```python
from build123d import *

# Parameters (mm, degrees)
F1_DEPTH = 38.1
F2_DEPTH = 2
F3_DEPTH = 12.7


with BuildPart() as f1:
    # F0 (on Top) → F1 (new body)
    with BuildSketch(Plane.XY):
        with BuildLine():
            Line((-57.138, -76.9493), (-18.130362, -76.9493))
            Line((-18.130362, -76.9493), (57.138, -76.9493))
            ThreePointArc((57.138, -76.9493), (71.1472, -71.1465), (76.95, -57.1373))
            Line((76.95, -57.1373), (76.95, 57.1373))
            ThreePointArc((76.95, 57.1373), (71.1472, 71.1465), (57.138, 76.9493))
            Line((57.138, 76.9493), (-57.138, 76.9493))
            ThreePointArc((-57.138, 76.9493), (-71.1472, 71.1465), (-76.95, 57.1373))
            Line((-76.95, 57.1373), (-76.95, -57.1373))
            ThreePointArc((-76.95, -57.1373), (-71.1472, -71.1465), (-57.138, -76.9493))
        make_face()
        with BuildLine():
            Line((-56.388, 76.2), (56.388, 76.2))
            ThreePointArc((56.388, 76.2), (70.3972, 70.3972), (76.2, 56.388))
            Line((76.2, 56.388), (76.2, -56.388))
            ThreePointArc((76.2, -56.388), (70.3972, -70.3972), (56.388, -76.2))
            Line((56.388, -76.2), (-18.130362, -76.2))
            Line((-18.130362, -76.2), (-56.388, -76.2))
            ThreePointArc((-56.388, -76.2), (-70.3972, -70.3972), (-76.2, -56.388))
            Line((-76.2, -56.388), (-76.2, 56.388))
            ThreePointArc((-76.2, 56.388), (-70.3972, 70.3972), (-56.388, 76.2))
        make_face(mode=Mode.SUBTRACT)
    extrude(amount=F1_DEPTH)

    # F0 (on Top) → F2 (join)
    with BuildSketch(Plane.XY):
        with BuildLine():
            ThreePointArc((76.2, 56.388), (70.3972, 70.3972), (56.388, 76.2))
            Line((56.388, 76.2), (-56.388, 76.2))
            ThreePointArc((-56.388, 76.2), (-70.3972, 70.3972), (-76.2, 56.388))
            Line((-76.2, 56.388), (-76.2, -56.388))
            ThreePointArc((-76.2, -56.388), (-70.3972, -70.3972), (-56.388, -76.2))
            Line((-56.388, -76.2), (-18.130362, -76.2))
            Line((-18.130362, -76.2), (56.388, -76.2))
            ThreePointArc((56.388, -76.2), (70.3972, -70.3972), (76.2, -56.388))
            Line((76.2, -56.388), (76.2, 56.388))
        make_face()
    extrude(amount=F2_DEPTH)

    # F0 (on Top) → F3 (join)
    with BuildSketch(Plane.XY):
        with BuildLine():
            Line((-57.138, -76.9493), (-18.130362, -76.9493))
            Line((-18.130362, -76.9493), (57.138, -76.9493))
            ThreePointArc((57.138, -76.9493), (71.1472, -71.1465), (76.95, -57.1373))
            Line((76.95, -57.1373), (76.95, 57.1373))
            ThreePointArc((76.95, 57.1373), (71.1472, 71.1465), (57.138, 76.9493))
            Line((57.138, 76.9493), (-57.138, 76.9493))
            ThreePointArc((-57.138, 76.9493), (-71.1472, 71.1465), (-76.95, 57.1373))
            Line((-76.95, 57.1373), (-76.95, -57.1373))
            ThreePointArc((-76.95, -57.1373), (-71.1472, -71.1465), (-57.138, -76.9493))
        make_face()
        with BuildLine():
            Line((-56.388, 76.2), (56.388, 76.2))
            ThreePointArc((56.388, 76.2), (70.3972, 70.3972), (76.2, 56.388))
            Line((76.2, 56.388), (76.2, -56.388))
            ThreePointArc((76.2, -56.388), (70.3972, -70.3972), (56.388, -76.2))
            Line((56.388, -76.2), (-18.130362, -76.2))
            Line((-18.130362, -76.2), (-56.388, -76.2))
            ThreePointArc((-56.388, -76.2), (-70.3972, -70.3972), (-76.2, -56.388))
            Line((-76.2, -56.388), (-76.2, 56.388))
            ThreePointArc((-76.2, 56.388), (-70.3972, 70.3972), (-56.388, 76.2))
        make_face(mode=Mode.SUBTRACT)
    extrude(amount=-F3_DEPTH)


solid = f1.part
```
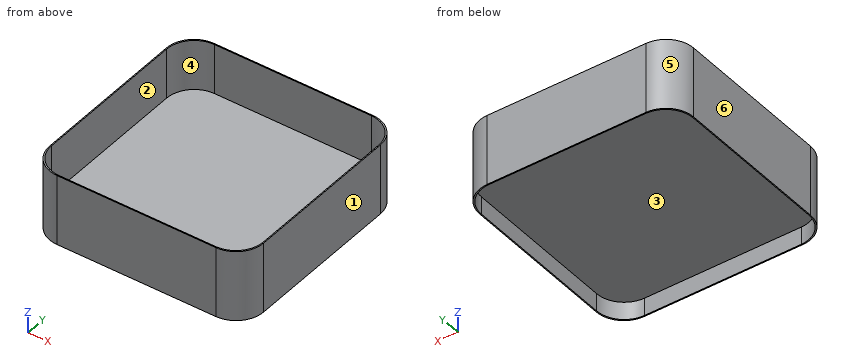
For this review, take the finished solid that the model builds, in its own axes (mm). Face numbers are marked on the shaded views. A direction names the side the tool comes from. Coordinates: 2 decimals unless noted, no trailing zeros. Write each loop counter-clockwise with the first axis right and the second up, starting at its lowest first coordinate (ties: lowest second). Pieces come first, ordered by that corner, then holes.
(1) Add section A-A on y = 10. Give the boundary of the cut face in (x, z), then the cut area to 3 significant figures.
(2) The part is to be moulded in two halves that separate along Y. For the marked faces 4, 5 and 6, say which applies: +Y half, -Y half, draft (parallel to the pull), parting line (faces both ways), or undercut.
(3) For pin 1 Ø6 at (x, y) = (-40, -37) entering from +Z, flat-tipped, find the tip position at first contact; note if it passes through.
(4) Wall thickness on probe 1 along Y at (x, z) = (42, 18.5); probe 2 along Z at (x, y) = (-48, -10.5): over which ranges is each line inside the solid? List them lowest first.
(5) Add section B-B on z = 24. Give the boundary of the cut face in (x, y).
(6) Tool access review of the marked faces 1, 2 and 3: name each direction out of +Z, -Z, +X, -X, +Y, -Y from which nothing blocks a thin tool from reaching the whole face with its end or side.
Answer sheet:
1. outline: (-76.95, -12.7) - (-76.2, -12.7) - (-76.2, 0) - (76.2, 0) - (76.2, -12.7) - (76.95, -12.7) - (76.95, 38.1) - (76.2, 38.1) - (76.2, 2) - (-76.2, 2) - (-76.2, 38.1) - (-76.95, 38.1) - close
1. area: 381 mm2
2. face 4: undercut
2. face 5: +Y half
2. face 6: draft
3. pin 1: stops at z = 2
4. probe 1: y = -76.95 to -76.2, 76.2 to 76.95
4. probe 2: z = 0 to 2
5. outline: (-76.95, -57.14) arc R19.81 ccw to (-57.14, -76.95) - (57.14, -76.95) arc R19.81 ccw to (76.95, -57.14) - (76.95, 57.14) arc R19.81 ccw to (57.14, 76.95) - (-57.14, 76.95) arc R19.81 ccw to (-76.95, 57.14) - close; hole (-76.2, -56.39) arc R19.81 ccw to (-56.39, -76.2) - (56.39, -76.2) arc R19.81 ccw to (76.2, -56.39) - (76.2, 56.39) arc R19.81 ccw to (56.39, 76.2) - (-56.39, 76.2) arc R19.81 ccw to (-76.2, 56.39) - close
6. face 1: +Z, -Z, +X, +Y, -Y
6. face 2: +Z
6. face 3: -Z
